Study the drawing (mm; zero at the part's minimum x, y, z) and answer. A direction names the side the tool comes from. Coordinates: 2 decimals unless noted, no trailing zeros. Loops run counter-clockwise (first coordinate to the right, second up) from the corner with the lowest first, then second, coordinate; pieces in that order, holes last. Notation, with made-up numbers: (55, 61) - (102, 61) arc R24 ccw to (102, 79) - close; hole circle Ø3 at (35, 37.5). An arc over 180 degrees is marked (long way). Use CSV: the item, a comma, the result in double quotes.
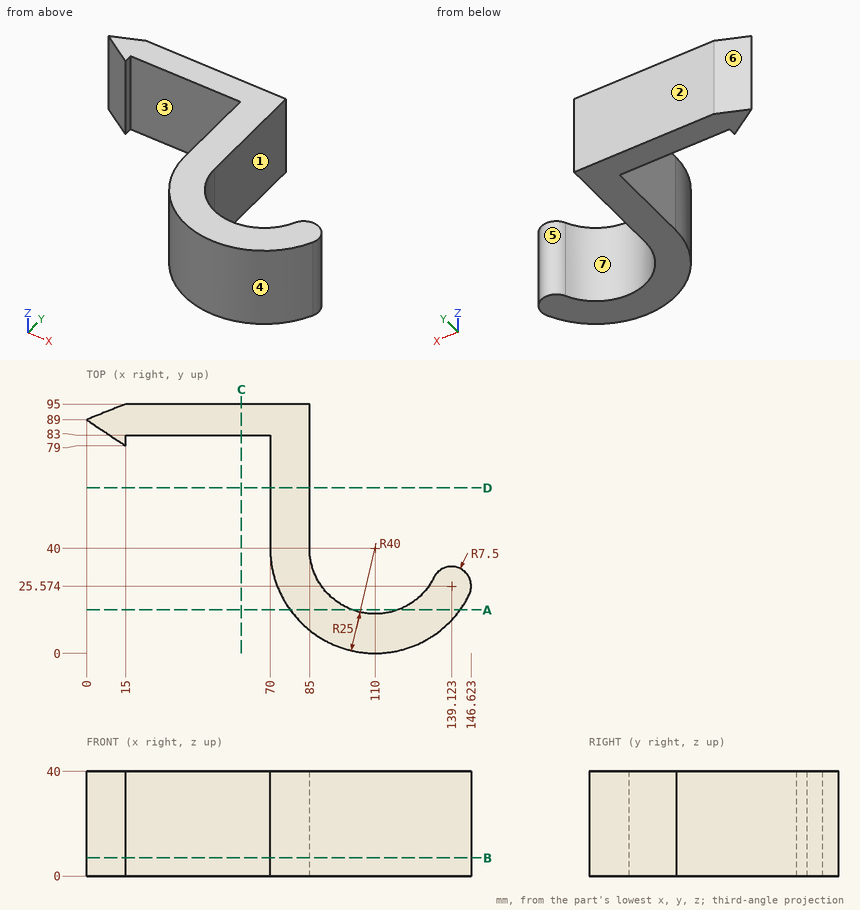
Q1. A tool of negligible diameter and unlimited length cuts with its end or side. For the marked faces 1, 2 and 3, from which of +Z, -Z, +X, -X, +Y, -Y can it reach the whole face along a straight path? Write none if from no direction.
Reported:
face 1,"+Z, -Z, +X, +Y"
face 2,"+Z, -Z, +X, -X, +Y"
face 3,"+Z, -Z, -Y"
Q2. The part is cut by section D-D on y = 63. Determine the outline of the cut face in (x, z), and give its area (3 significant figures).
Reported:
outline,"(70, 0) - (85, 0) - (85, 40) - (70, 40) - close"
area,"600 mm²"
Q3. The part is cut by section B-B on z = 7. Determine the outline of the cut face in (x, y) (1 decimal).
Reported:
outline,"(0, 89) - (15, 79) - (15, 83) - (70, 83) - (70, 40) arc R40 ccw to (145.8, 22.2) arc R7.5 ccw to (132.4, 28.9) arc R25 cw to (85, 40) - (85, 95) - (15, 95) - close"
Q4. The part is cut by section A-A on y = 16.5. Determine the outline of the cut face in (x, z).
Reported:
outline,"(77.63, 0) - (101.47, 0) - (101.47, 40) - (77.63, 40) - close; (118.53, 0) - (142.37, 0) - (142.37, 40) - (118.53, 40) - close"
Q5. Find the intervals of material crossed by probe 1 along Y at (x, z) = (29, 11.5); probe 2 along X at (y, z) = (78, 32); probe 3 along X at (y, z) = (29.5, 17.5) (1 decimal), in increasing order. Write a range as [from, to].
Reported:
probe 1,"y = [83, 95]"
probe 2,"x = [70, 85]"
probe 3,"x = [71.4, 87.3], [132.7, 145.5]"
Q6. The part is cut by section C-C on x = 59. Determine the outline of the cut face in (y, z), and give its area (3 significant figures).
Reported:
outline,"(83, 0) - (95, 0) - (95, 40) - (83, 40) - close"
area,"480 mm²"
Q7. Given P1, Ø4, axis at y = 15, z = 29, coming from the +X side (1 decimal); P2, Ø20, axis at y = 56, z = 16.5, coming from the -X side; P3, Ø4.5, axis at y = 81, z = 19.5, coming from the +X side, each flat-ended and moving along its own axis, determine where each tip first touches the part or whether it passes through.
Reported:
P1,"stops at x = 142.7"
P2,"stops at x = 70"
P3,"stops at x = 85"
Q8. For a pull along X with two mould halves and no side action, classify the marked faces 4, 5, 6 and 7 as +X half, -X half, draft (parallel to the pull), parting line (faces both ways), or undercut.
Reported:
face 4,"parting line"
face 5,"undercut"
face 6,"-X half"
face 7,"undercut"
